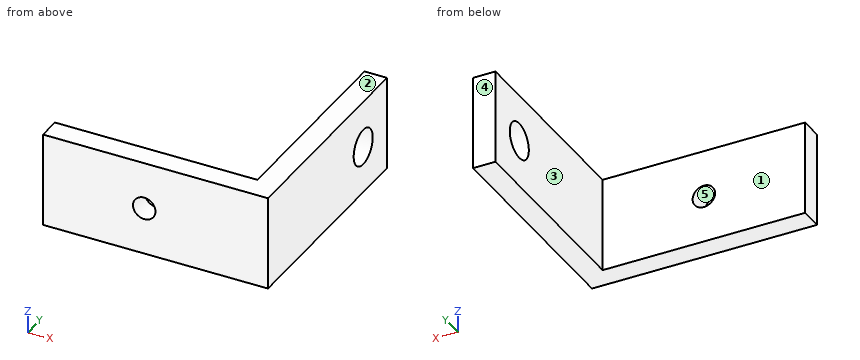
from build123d import *

# Parameters (mm, degrees)
BOSS_EXTRUDE1_DEPTH = 21
SKETCH3_R           = 4
CUT_EXTRUDE1_DEPTH  = 71.46985171
SKETCH4_R           = 2.5
CUT_EXTRUDE2_DEPTH  = 74.763134424


with BuildPart() as part:
    # Sketch2 → Boss-Extrude1 (new body)
    with BuildSketch(Plane.XY):
        Polygon((0, 0), (0, 50), (-5, 50), (-5, 5), (-50, 5), (-50, 0), align=None)
    extrude(amount=BOSS_EXTRUDE1_DEPTH)

    # Sketch3 → Cut-Extrude1 (cut, through all)
    with BuildSketch(Plane.ZY.offset(5)):
        with Locations(Location((10.5, 40, 0), (0, 0, 270))):
            Circle(SKETCH3_R)
    extrude(amount=-CUT_EXTRUDE1_DEPTH, mode=Mode.SUBTRACT)

    # Sketch4 → Cut-Extrude2 (cut, through all)
    with BuildSketch(Plane(origin=(0, 0, 0), x_dir=(1, 0, 0), z_dir=(0, 1, 0))):
        with Locations((-27.5, -10.5)):
            Circle(SKETCH4_R)
    extrude(amount=CUT_EXTRUDE2_DEPTH, mode=Mode.SUBTRACT)


solid = part.part
For this review, take the finished solid that the model builds, in its own axes (mm). Face numbers are marked on the shaded views. A direction names the side the tool comes from. Round coordinates to 2 decimals unless told otherwise and drop trailing zeros. Loops run counter-clockwise (first coordinate to the right, second up) from the corner with the lowest first, then second, coordinate; pieces in that order, holes last. Notation, with made-up numbers: (57, 15.25) - (81, 15.25) arc R13 cw to (81, 19.25) - close; hole circle Ø3 at (-23.5, 84). An arc over 180 degrees is marked (long way). One line per item, written item: value. Start each with the question number.
Item 1: Take a section at C-C (x = -27.5). Give the boundary of the cut face in (y, z), plus the area to 3 significant figures.
Item 2: Take a section at B-B (y = 40). Give the boundary of the cut face in (x, z).
Item 3: Clearance check with flat-ended pins moving along their axes: pin 1 Ø8 at (x, z) = (-27.5, 10.5) entering from +Y; pin 2 Ø1.5 at (x, z) = (-38, 15) entering from -Y; pin 3 Ø5 at (y, z) = (38.5, 12.5) entering from -X. State where each tip first meets the part, or that it passes through.
Item 4: For L1, parallel to Z at x = -1.15, y = 40; L2, parallel to X at y = 3.9, z = 10.5; L3, parallel to Y at x = -44, z = 19.5, list the stretches that pass through material, from the lowest coordinate up.
Item 5: The part is to be moulded in two halves that separate along X. For the marked faces 3, 4 and 5, say which applies: +X half, -X half, draft (parallel to the pull), parting line (faces both ways), or undercut.
Item 6: Take a section at A-A (z = 10.5). Give the boundary of the cut face in (x, y).
Item 7: Take a section at D-D (z = 5.25). Give the boundary of the cut face in (x, y).
Item 8: For the marked faces 1 and 2, list the 3-axis set-ups (+Z, -Z, +X, -X, +Y, -Y) from which the entire face can be reached by the end or side of a thin tool; tool diameter is ignored.
Answer below:
1. outline: (0, 0) - (5, 0) - (5, 8) - (0, 8) - close; (0, 13) - (5, 13) - (5, 21) - (0, 21) - close
1. area: 80.0 mm2
2. outline: (-5, 0) - (0, 0) - (0, 6.5) - (-5, 6.5) - close; (-5, 14.5) - (0, 14.5) - (0, 21) - (-5, 21) - close
3. pin 1: stops at y = 5
3. pin 2: stops at y = 0
3. pin 3: stops at x = -5
4. L1: z = 0 to 6.5, 14.5 to 21
4. L2: x = -50 to -30, -25 to 0
4. L3: y = 0 to 5
5. face 3: -X half
5. face 4: draft
5. face 5: undercut
6. outline: (-50, 0) - (-30, 0) - (-30, 5) - (-50, 5) - close; (-25, 0) - (0, 0) - (0, 36) - (-5, 36) - (-5, 5) - (-25, 5) - close; (-5, 44) - (0, 44) - (0, 50) - (-5, 50) - close
7. outline: (-50, 0) - (0, 0) - (0, 50) - (-5, 50) - (-5, 5) - (-50, 5) - close
8. face 1: +Z, -Z, -X, +Y
8. face 2: +Z, +X, -X, +Y, -Y
